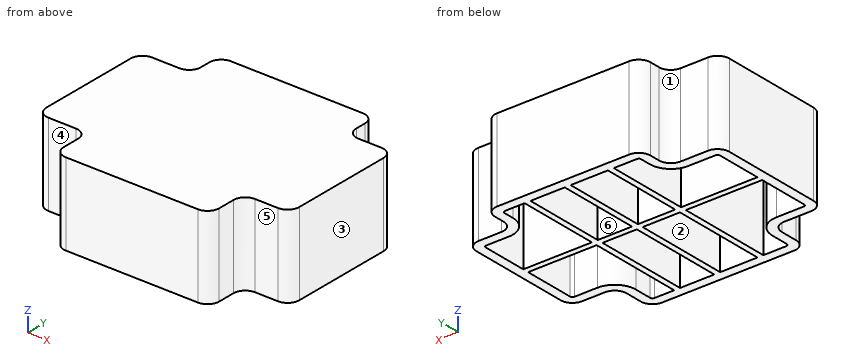
from build123d import *

# Parameters (mm, degrees)
BOSS_EXTRUDE1_DEPTH = 70
SHELL1_T            = -8
RIB15_REACH         = 159.422
SKETCH3_WALLS_W     = 5
SKETCH3_WALLS_H     = 472.061491267
SKETCH3_WALLS_W_2   = 516.540635297
SKETCH3_WALLS_H_2   = 5


with BuildPart() as part:
    # Sketch1 → Boss-Extrude1 (new body)
    with BuildSketch(Plane.XY):
        with BuildLine():
            Line((76.31679607, 53.723303483), (95.972900387, 53.723303483))
            ThreePointArc((95.972900387, 53.723303483), (103.043968199, 50.794371295), (105.972900387, 43.723303483))
            Line((105.972900387, 43.723303483), (105.972900387, -43.723303483))
            ThreePointArc((105.972900387, -43.723303483), (103.043968199, -50.794371295), (95.972900387, -53.723303483))
            Line((95.972900387, -53.723303483), (76.31679607, -53.723303483))
            ThreePointArc((76.31679607, -53.723303483), (69.245728258, -56.652235671), (66.31679607, -63.723303483))
            Line((66.31679607, -63.723303483), (66.31679607, -78.556368085))
            ThreePointArc((66.31679607, -78.556368085), (63.387863882, -85.627435897), (56.31679607, -88.556368085))
            Line((56.31679607, -88.556368085), (-56.31679607, -88.556368085))
            ThreePointArc((-56.31679607, -88.556368085), (-63.387863882, -85.627435897), (-66.31679607, -78.556368085))
            Line((-66.31679607, -78.556368085), (-66.31679607, -63.723303483))
            ThreePointArc((-66.31679607, -63.723303483), (-69.245728258, -56.652235671), (-76.31679607, -53.723303483))
            Line((-76.31679607, -53.723303483), (-99.724153498, -53.723303483))
            ThreePointArc((-99.724153498, -53.723303483), (-106.79522131, -50.794371295), (-109.724153498, -43.723303483))
            Line((-109.724153498, -43.723303483), (-109.724153498, 43.723303483))
            ThreePointArc((-109.724153498, 43.723303483), (-106.79522131, 50.794371295), (-99.724153498, 53.723303483))
            Line((-99.724153498, 53.723303483), (-76.31679607, 53.723303483))
            ThreePointArc((-76.31679607, 53.723303483), (-69.245728258, 56.652235671), (-66.31679607, 63.723303483))
            Line((-66.31679607, 63.723303483), (-66.31679607, 72.661541768))
            ThreePointArc((-66.31679607, 72.661541768), (-63.387863882, 79.73260958), (-56.31679607, 82.661541768))
            Line((-56.31679607, 82.661541768), (56.31679607, 82.661541768))
            ThreePointArc((56.31679607, 82.661541768), (63.387863882, 79.73260958), (66.31679607, 72.661541768))
            Line((66.31679607, 72.661541768), (66.31679607, 63.723303483))
            ThreePointArc((66.31679607, 63.723303483), (69.245728258, 56.652235671), (76.31679607, 53.723303483))
        make_face()
    extrude(amount=BOSS_EXTRUDE1_DEPTH)

    # Shell1
    shell1_openings = [part.faces().sort_by_distance(p)[0] for p in [
        (-1.372763961, -2.113601646, 0),
    ]]
    offset(amount=SHELL1_T, openings=shell1_openings, kind=Kind.INTERSECTION)

    # Sketch3 walls → Rib15 (add, up to next)
    with BuildSketch(Plane.XY, mode=Mode.PRIVATE) as rib15_sk1:
        with Locations((-34.103750382, -2.947413158)):
            Rectangle(SKETCH3_WALLS_W, SKETCH3_WALLS_H)
    rib15_tool1 = extrude(rib15_sk1.sketch, amount=RIB15_REACH, mode=Mode.PRIVATE) - part.part
    # Sketch3 walls → Rib15 (add, up to next)
    with BuildSketch(Plane.XY, mode=Mode.PRIVATE) as rib15_sk2:
        with Locations((2.728391134, -2.947413158)):
            Rectangle(SKETCH3_WALLS_W, SKETCH3_WALLS_H)
    rib15_tool2 = extrude(rib15_sk2.sketch, amount=RIB15_REACH, mode=Mode.PRIVATE) - part.part
    # Sketch3 walls → Rib15 (add, up to next)
    with BuildSketch(Plane.XY, mode=Mode.PRIVATE) as rib15_sk3:
        with Locations((36.963394466, -2.947413158)):
            Rectangle(SKETCH3_WALLS_W, SKETCH3_WALLS_H)
    rib15_tool3 = extrude(rib15_sk3.sketch, amount=RIB15_REACH, mode=Mode.PRIVATE) - part.part
    # Sketch3 walls → Rib15 (add, up to next)
    with BuildSketch(Plane.XY, mode=Mode.PRIVATE) as rib15_sk4:
        with Locations((-1.875626555, 2.364914945)):
            Rectangle(SKETCH3_WALLS_W_2, SKETCH3_WALLS_H_2)
    rib15_tool4 = extrude(rib15_sk4.sketch, amount=RIB15_REACH, mode=Mode.PRIVATE) - part.part
    add(rib15_tool1.solids().sort_by_distance((-34.103750382, -2.947413159, 0))[0])
    add(rib15_tool2.solids().sort_by_distance((2.728391134, -2.947413159, 0))[0])
    add(rib15_tool3.solids().sort_by_distance((36.963394466, -2.947413159, 0))[0])
    add(rib15_tool4.solids().sort_by_distance((-1.875626556, 2.364914945, 0))[0])


solid = part.part
Build history of the part. All positions in model axes, mm. Face numbers are marked on the shaded views. A direction names the side the tool comes from. Coordinates: 2 decimals unless noted, no trailing zeros. Write each loop counter-clockwise with the first axis right and the second up, starting at its lowest first coordinate (ties: lowest second). Pieces come first, ordered by that corner, then holes. Notation, with made-up numbers: (21, 28) -> (35, 28) arc R31 cw to (35, 66) -> close; hole circle Ø4 at (17, 15.5). An arc over 180 degrees is marked (long way). Use CSV: the item, a comma, the result in double quotes. Start each with the question number.
Q1. Cut at A-A, the plane x = -39. List the corners of the cut face in (y, z), then the cut area to 3 significant figures.
Q2. Cut at C-C, the plane z = 38. State how many separate pieces and enclosed holes the cut face has, then the cut area to 3 significant figures.
Q3. 3-axis set-ups, long thin cutter, end or side, ignore diameter. For the marked faces 4, 5 and 6: which of +Z, -Z, +X, -X, +Y, -Y reach the whole face in a straight line?
Q4. Pull direction X, two halves, no side cores. Call the marked faces 1, 2 and 3: released by +X, released by -X, zero draft, split by the parting line, or undercut.
Q5. Cut at D-D, the plane x = 87.5. List the corners of the cut face in (y, z).
Q6. Flat gauge pins, fed straight in: pin 1 Ø8 at (x, z) = (-82, 63) entering from -Y; pin 2 Ø3 at (y, z) = (-66, 39) entering from +X; pin 3 Ø18.5 at (x, z) = (-88, 17.5) entering from +Y. Where does each tip first touch, or does it go through?
Q7. Cut at B-B, the plane y = -39.5. List the corners of the cut face in (x, z), then the cut area to 3 significant figures.
Q8. Drill centre lines: probe 1 along X at (y, z) = (68.5, 30.5); probe 2 along Y at (x, z) = (52, 51); probe 3 along X at (y, z) = (-28, 22). Where is each one in solid material? Low to high.
Checked values:
1,outline,"(-88.56, 0) -> (-80.56, 0) -> (-80.56, 62) -> (-0.14, 62) -> (-0.14, 0) -> (4.86, 0) -> (4.86, 62) -> (74.66, 62) -> (74.66, 0) -> (82.66, 0) -> (82.66, 70) -> (-88.56, 70) -> close"
1,area,"2,670 mm²"
2,separate pieces,"1"
2,enclosed holes,"8"
2,area,"8,830 mm²"
3,face 4,"+Z, -Z, -X, -Y"
3,face 5,"+Z, -Z, +X, -Y"
3,face 6,"-Z"
4,face 1,"released by -X"
4,face 2,"undercut"
4,face 3,"released by +X"
5,outline,"(-53.72, 0) -> (-45.72, 0) -> (-45.72, 62) -> (-0.14, 62) -> (-0.14, 0) -> (4.86, 0) -> (4.86, 62) -> (45.72, 62) -> (45.72, 0) -> (53.72, 0) -> (53.72, 70) -> (-53.72, 70) -> close"
6,pin 1,"stops at y = -53.72"
6,pin 2,"stops at x = 66.32"
6,pin 3,"stops at y = 53.72"
7,outline,"(-109.72, 0) -> (-101.72, 0) -> (-101.72, 62) -> (-36.6, 62) -> (-36.6, 0) -> (-31.6, 0) -> (-31.6, 62) -> (0.23, 62) -> (0.23, 0) -> (5.23, 0) -> (5.23, 62) -> (34.46, 62) -> (34.46, 0) -> (39.46, 0) -> (39.46, 62) -> (97.97, 62) -> (97.97, 0) -> (105.97, 0) -> (105.97, 70) -> (-109.72, 70) -> close"
7,area,"3,650 mm²"
8,probe 1,"x = -66.32 to -58.32, -36.6 to -31.6, 0.23 to 5.23, 34.46 to 39.46, 58.32 to 66.32"
8,probe 2,"y = -88.56 to -80.56, -0.14 to 4.86, 74.66 to 82.66"
8,probe 3,"x = -109.72 to -101.72, -36.6 to -31.6, 0.23 to 5.23, 34.46 to 39.46, 97.97 to 105.97"
